Can you work these out from the model? Positions are in its coordinate system, mm. A direction names the side the tool comes from. Give positions to 0.01 mm unless a question says otherwise; leave off trailing zeros. Loops run counter-clockwise (first coordinate to the right, second up) from the corner with the lowest first, then second, coordinate; pieces in that order, holes last. Notation, with made-up numbers: (-28, -19) -> (26, -19) arc R16 ccw to (26, -9) -> close; hole circle Ø10 at (0, -13). An arc over 180 degrees is marked (long way). Use CSV: the item, a comma, the result in double quotes.
from build123d import *

# Parameters (mm, degrees)
F1_DEPTH = 20
F2_R     = 5
F2_W     = 4
F2_H     = 5
F3_DEPTH = 2.001
F4_R     = 5
F5_DEPTH = 2.001
F6_R     = 3
F7_R     = 1


with BuildPart() as f1:
    # F0 (on Right) → F1 (new body)
    with BuildSketch(Plane.YZ):
        Polygon((0, 2), (0, 0), (30, 0), (30, 30), (28, 30), (28, 2), align=None)
    extrude(amount=F1_DEPTH)

    # F2 (on face) → F3 (cut, through all)
    with BuildSketch(Plane.XZ.offset(-28)):
        with Locations((10, 20)):
            Circle(F2_R)
        with Locations((18, 7.5)):
            Rectangle(F2_W, F2_H)
    extrude(amount=-F3_DEPTH, mode=Mode.SUBTRACT)

    # F4 (on face) → F5 (cut, through all)
    with BuildSketch(Plane.XY.offset(2)):
        with Locations((10, 10)):
            Circle(F4_R)
    extrude(amount=-F5_DEPTH, mode=Mode.SUBTRACT)

    # F6
    f6_edges = [f1.edges().sort_by_distance(p)[0] for p in [
        (10, 28, 2),
        (10, 30, 0),
    ]]
    fillet(f6_edges, radius=F6_R)

    # F7
    f7_edges = [f1.edges().sort_by_distance(p)[0] for p in [
        (0, 0, 1),
        (20, 0, 1),
        (20, 29, 30),
        (0, 29, 30),
    ]]
    fillet(f7_edges, radius=F7_R)


solid = f1.part
(1) If I drill on L1, parallel to Z at x = 13.5, y = 14.5; L2, parallel to Y at x = 6, z = 24; L3, parallel to X at y = 28.5, z = 6.5, over which ranges is the centre line in solid material (lowest first)? Write a range as from..to.
Answer sheet:
L1,"z = 0..2"
L2,"y = 28..30"
L3,"x = 0..16"
(2) If we section it at B-B, the plane z = 20: Write out the boundary of the cut face in (x, y).
Answer sheet:
outline,"(0, 28) -> (5, 28) -> (5, 30) -> (0, 30) -> close; (15, 28) -> (20, 28) -> (20, 30) -> (15, 30) -> close"
(3) If we section it at A-A, the plane y = 10: Write out the boundary of the cut face in (x, z).
Answer sheet:
outline,"(0, 0) -> (5, 0) -> (5, 2) -> (0, 2) -> close; (15, 0) -> (20, 0) -> (20, 2) -> (15, 2) -> close"
(4) If we section it at D-D, the plane x = 10: Write out the boundary of the cut face in (y, z), then the cut area to 3 significant figures.
Answer sheet:
outline,"(0, 0) -> (5, 0) -> (5, 2) -> (0, 2) -> close; (15, 0) -> (27, 0) arc R3 ccw to (30, 3) -> (30, 15) -> (28, 15) -> (28, 5) arc R3 cw to (25, 2) -> (15, 2) -> close; (28, 25) -> (30, 25) -> (30, 30) -> (28, 30) -> close"
area,"76.0 mm2"
(5) Will these pins go through, and if not, where does the flat tip stop? pin 1 Ø1 at (x, y) = (16, 17) entering from +Z; pin 2 Ø1 at (x, y) = (18.5, 29.5) entering from -Z; pin 3 Ø1.5 at (x, z) = (16.5, 9) entering from -Y; pin 4 Ø6 at (x, z) = (10, 20) entering from -Y.
Answer sheet:
pin 1,"stops at z = 2"
pin 2,"stops at z = 0.76"
pin 3,"stops at y = 28"
pin 4,"passes through"
(6) We'd pull the mould along Z, two halves only. Please class faces 4 (the face through (20, 29, 20)), 5 (the face through (10, 29, 30)), 6 (the face through (18, 29, 10)): released by +Z, released by -Z, zero draft, split by the parting line, or undercut.
Answer sheet:
face 4,"zero draft"
face 5,"released by +Z"
face 6,"undercut"
(7) If we section it at C-C, the plane x = 18.25: Write out the boundary of the cut face in (y, z).
Answer sheet:
outline,"(0, 0) -> (27, 0) arc R3 ccw to (30, 3) -> (30, 5) -> (28, 5) arc R3 cw to (25, 2) -> (0, 2) -> close; (28, 10) -> (30, 10) -> (30, 30) -> (28, 30) -> close"
(8) Which directions (+Z, -Z, +X, -X, +Y, -Y) give clear straight access to the entire face, cutting with the end or side of a thin tool? Please do faces 1 (the face through (18, 29, 5)), 2 (the face through (8, 28, 15)), 3 (the face through (12.307, 28.986, 15.564)).
Answer sheet:
face 1,"+X, +Y, -Y"
face 2,"+Z, +X, -X, -Y"
face 3,"+Y, -Y"
